from build123d import *

# Parameters (mm, degrees)
SKETCH_2_R             = 1.5
EXTRUDE_1_DEPTH        = 2
HOLE_WIZARD_M3_2_D     = 2.5
HOLE_WIZARD_M3_2_DEPTH = 6
HOLE_WIZARD_M3_2_TIP   = 0.751075774
CUT_EXTRUDE_1_DEPTH    = 5
EXTRUDE_2_DEPTH        = 14


with BuildPart() as part:
    # 草图1 → 旋转1 (revolve)
    with BuildSketch(Plane.XY):
        Polygon((0, 0), (0, 16), (12, 16), (12, 13), (14, 13), (14, 12.25), (25.2, 12.25), (25.2, 0), align=None)
    revolve(axis=Axis((25.2, 0, 0), (-1, 0, 0)))

    # 草图2 → 凸台-拉伸1 (add)
    with BuildSketch(Plane.ZY):
        with BuildLine():
            Line((4, 19.5), (4, -19.5))
            ThreePointArc((4, -19.5), (0, -23.5), (-4, -19.5))
            Line((-4, -19.5), (-4, 19.5))
            ThreePointArc((-4, 19.5), (0, 23.5), (4, 19.5))
        make_face()
        with Locations(Location((0, 19.5, 0), (0, 0, 270))):
            Circle(SKETCH_2_R, mode=Mode.SUBTRACT)
        with Locations(Location((0, -19.5, 0), (0, 0, 270))):
            Circle(SKETCH_2_R, mode=Mode.SUBTRACT)
    extrude(amount=-EXTRUDE_1_DEPTH)

    # 草图4 → 旋转2 (revolve)
    with BuildSketch(Plane.XY.offset(-8), mode=Mode.PRIVATE) as revolve_2_sk:
        Polygon((0, 0), (0, 4.25), (-0.5, 4.25), (-0.5, 4), (-2.7, 4), (-2.7, 2.5), (-10.2, 2.5), (-10.2, 0), align=None)
    revolve(revolve_2_sk.sketch.rotate(Axis((-10.2, 0, -8), (1, 0, 0)), 180), axis=Axis((-10.2, 0, -8), (1, 0, 0)))

    # M3 螺纹孔2
    with Locations(Plane.ZY.offset(10.2)):
        with Locations((-8, 0)):
            Hole(HOLE_WIZARD_M3_2_D / 2, depth=HOLE_WIZARD_M3_2_DEPTH)
            with Locations((0, 0, -(HOLE_WIZARD_M3_2_DEPTH + HOLE_WIZARD_M3_2_TIP / 2))):  # 118° drill point
                Cone(0, HOLE_WIZARD_M3_2_D / 2, HOLE_WIZARD_M3_2_TIP, mode=Mode.SUBTRACT)

    # 草图5 → 切除-拉伸1 (cut)
    with BuildSketch(Plane.ZY.offset(10.2)):
        with BuildLine():
            Line((-10, -1.5), (-10, 1.5))
            ThreePointArc((-10, 1.5), (-10.5, 0), (-10, -1.5))
        make_face()
        with BuildLine():
            ThreePointArc((-5.5, 0), (-5.628291755, 0.790569415), (-6, 1.5))
            Line((-6, 1.5), (-6, -1.5))
            ThreePointArc((-6, -1.5), (-5.628291755, -0.790569415), (-5.5, 0))
        make_face()
    extrude(amount=-CUT_EXTRUDE_1_DEPTH, mode=Mode.SUBTRACT)

    # 草图9 → 凸台-拉伸2 (add)
    with BuildSketch(Plane.XY):
        with BuildLine():
            Line((24.75, 2.995850319), (24.75, -3.004149681))
            ThreePointArc((24.75, -3.004149681), (24, -3.754149681), (23.25, -3.004149681))
            Line((23.25, -3.004149681), (23.25, 2.995850319))
            ThreePointArc((23.25, 2.995850319), (24, 3.745850319), (24.75, 2.995850319))
        make_face()
    extrude(amount=EXTRUDE_2_DEPTH)


solid = part.part
CAD build for the part. Positions are in the model's coordinates, mm. A direction names the side the tool comes from. Round coordinates to 2 decimals unless told otherwise and drop trailing zeros. Write each loop counter-clockwise with the first axis right and the second up, starting at its lowest first coordinate (ties: lowest second). Pieces come first, ordered by that corner, then holes. Notation, with made-up numbers: M 78.5,17.5 L 103.5,17.5 A11 cw 103.5,25.5 Z; hole C 72,32 d6. An arc over 180 degrees is marked long. Put each result on its own line as item: value. Start each with the question number.
1) 3-axis set-ups, long thin cutter, end or side, ignore diameter. For faces 5 (the flat face through (1, -17, 4)), 6 (the cylindrical face through (23.984, 3.746, 12.815)), 7 (the flat face through (1, 18, 4)), 8 (the flat face through (-8, 0, -10)), 9 (the flat face through (-8, 0, -6)): which of +Z, -Z, +X, -X, +Y, -Y reach the whole face in a straight line?
2) Saw through at C-C, the plane x = 24. Write the cut outline in (y, z).
3) Pull direction Y, two halves, no side cores. Call faces 1 (the conical face through (-3.579, -0.132, -8.172)), 2 (the flat face through (0, 0, 0)), 3 (the cylindrical face through (19.678, 6.586, -10.329)), 4 (the cylindrical face through (24.016, -3.754, 12.814)): pulls with the +Y half, pulls with the -Y half, needs draft (parallel to the pull), parting line crosses it, or undercut.
4) Drill centre lines: probe 1 along Z at (x, y) = (1.3, 19.5); probe 2 along Z at (x, y) = (-8.9, 0); probe 3 along X at (y, z) = (-11, -11.5). Where is each one in solid material? Low to high. Write a range as [from, to].
5) Saw through at B-B, the plane x = -7. Write the cut outline in (y, z).
6) Pin check, flat tips, straight feed: pin 1 Ø2.5 at (x, y) = (-8.5, 0) entering from -Z; pin 2 Ø2.5 at (x, y) = (-7, 0.5) entering from +Z; pin 3 Ø10 at (x, y) = (14.5, -10.5) entering from +Z; pin 4 Ø3 at (y, z) = (0, -8) entering from -X. Stop position of each tip, or through.
7) Saw through at A-A, the plane z = 0. Write the cut outline in (x, y).
8) Saw through at D-D, the plane y = 5. Write the cut outline in (x, z), and give its area (3 significant figures).
Resolved:
1. face 5: +Z, +X, -X, -Y
1. face 6: +Z, +Y
1. face 7: +Z, +X, -X, +Y
1. face 8: -Z, -X, +Y, -Y
1. face 9: +Z, -X, +Y, -Y
2. outline: M -3.75,11.66 A12.25 ccw long 3.75,11.66 L 3.75,14 L -3.75,14 Z
3. face 1: undercut
3. face 2: needs draft
3. face 3: parting line crosses it
3. face 4: pulls with the -Y half
4. probe 1: [-4, -1.5], [1.5, 4]
4. probe 2: [-10, -9.25], [-6.75, -6]
4. probe 3: [0, 12]
5. outline: M -1.5,-10 L 1.5,-10 A2.5 ccw 1.5,-6 L -1.5,-6 A2.5 ccw Z; hole C 0,-8 d2.5
6. pin 1: z = -10
6. pin 2: z = -6
6. pin 3: z = 14.76
6. pin 4: x = -10.2
7. outline: M 0,-23.5 L 2,-23.5 L 2,-21 L 0,-21 Z; M 0,-18 L 2,-18 L 2,-16 L 12,-16 L 12,-13 L 14,-13 L 14,-12.25 L 25.2,-12.25 L 25.2,12.25 L 14,12.25 L 14,13 L 12,13 L 12,16 L 2,16 L 2,18 L 0,18 Z; M 0,21 L 2,21 L 2,23.5 L 0,23.5 Z
8. outline: M 0,-15.2 L 12,-15.2 L 12,-12 L 14,-12 L 14,-11.18 L 25.2,-11.18 L 25.2,11.18 L 14,11.18 L 14,12 L 12,12 L 12,15.2 L 0,15.2 Z
8. area: 663 mm²
